from build123d import *

# Parameters (mm, degrees)
SKETCH1_R                = 7.5
BOSS_EXTRUDE1_DEPTH      = 8
M4_CLEARANCE_HOLE1_D     = 4.3
M4_CLEARANCE_HOLE1_DEPTH = 25
M4_CLEARANCE_HOLE1_TIP   = 1.291850331


with BuildPart() as part:
    # Sketch1 → Boss-Extrude1 (new body)
    with BuildSketch(Plane.XY):
        with BuildLine():
            Line((0.318181818, 17.497107199), (110.281818182, 15.497437805))
            ThreePointArc((110.281818182, 15.497437805), (125.5, 0), (110.281818182, -15.497437805))
            Line((110.281818182, -15.497437805), (0.318181818, -17.497107199))
            ThreePointArc((0.318181818, -17.497107199), (-17.5, 0), (0.318181818, 17.497107199))
        make_face()
        with Locations((110, 0)):
            Circle(SKETCH1_R, mode=Mode.SUBTRACT)
        with BuildLine():
            Line((35, 6.828401482), (35, -6.828401482))
            ThreePointArc((35, -6.828401482), (35.598701901, -8.255413618), (37.036363636, -8.828070876))
            Line((37.036363636, -8.828070876), (83.036363636, -7.991568964))
            ThreePointArc((83.036363636, -7.991568964), (84.427012136, -7.393197669), (85, -5.991899569))
            Line((85, -5.991899569), (85, 5.991899569))
            ThreePointArc((85, 5.991899569), (84.427012136, 7.393197669), (83.036363636, 7.991568964))
            Line((83.036363636, 7.991568964), (37.036363636, 8.828070876))
            ThreePointArc((37.036363636, 8.828070876), (35.598701901, 8.255413618), (35, 6.828401482))
        make_face(mode=Mode.SUBTRACT)
    extrude(amount=BOSS_EXTRUDE1_DEPTH)

    # M4 Clearance Hole1
    with Locations(Plane.XY.offset(8)):
        with Locations((12.124355653, 7), (0, 14), (-12.124355653, 7), (-12.124355653, -7), (0, -14), (12.124355653, -7)):
            Hole(M4_CLEARANCE_HOLE1_D / 2, depth=M4_CLEARANCE_HOLE1_DEPTH)
            with Locations((0, 0, -(M4_CLEARANCE_HOLE1_DEPTH + M4_CLEARANCE_HOLE1_TIP / 2))):  # 118° drill point
                Cone(0, M4_CLEARANCE_HOLE1_D / 2, M4_CLEARANCE_HOLE1_TIP, mode=Mode.SUBTRACT)


solid = part.part
Could you check a few things on this model? Use its own coordinates, in mm. A direction names the side the tool comes from. Give positions to 0.01 mm unless a question says otherwise; leave off trailing zeros. Order: outer loops, then holes, each group sorted by start corner. A loop starts at its lowest first (then second) coordinate and runs counter-clockwise, first axis right, second up.
1. For faces 5 (the flat face through (55, -11, 0)), 6 (the flat face through (35, 0, 4)), which set-ups out of +Z, -Z, +X, -X, +Y, -Y let a thin tool reach every point of the face, with its end or its side?
2. I need wall thicknesses on L1, parallel to Y at x = 14, z = 5; L2, parallel to Y at x = 13, z = 6; L3, parallel to X at y = -1, z = 2. Which ranges of each line are inside material? Lowest first, please.
3. We'd pull the mould along Y, two halves only. Please class faces 1 (the flat face through (55, -11, 8)), 2 (the cylindrical face through (-11.84, -4.87, 3.94)), 3 (the cylindrical face through (-17.496, -0.389, 3.944)), 4 (the cylindrical face through (0.47, 11.9, 3.94)): pulls with the +Y half, pulls with the -Y half, needs draft (parallel to the pull), parting line crosses it, or undercut.
4. Suppose I cut it at D-D (y = -14). List the corners of the cut face in (x, z) for me.
5. Will these pins go through, and if not, where does the flat tip stop? P1, Ø1, axis at x = 16, z = 6, coming from the +Y side; P2, Ø4, axis at y = 10.5, z = 1.5, coming from the +X side.
6. Suppose I cut it at B-B (z = 5.25). Give the number of separate pieces and of enclosed holes in the cut face, plus the area to 3 significant figures.
7. Suppose I cut it at C-C (x = 76). List the corners of the cut face in (y, z) for me, plus the area to 3 significant figures.
8. Suppose I cut it at A-A (y = 0). List the corners of the cut face in (x, z) for me.
Solved:
1. face 5: -Z, +X, -X, +Y, -Y
1. face 6: +Z, -Z
2. L1: y = -17.25 to -8.05, -5.95 to 5.95, 8.05 to 17.25
2. L2: y = -17.27 to -8.96, -5.04 to 5.04, 8.96 to 17.27
2. L3: x = -17.47 to 35, 85 to 102.57, 117.43 to 125.47
3. face 1: needs draft
3. face 2: undercut
3. face 3: parting line crosses it
3. face 4: undercut
4. outline: (-10.5, 0) - (-2.15, 0) - (-2.15, 8) - (-10.5, 8) - close; (2.15, 0) - (116.65, 0) - (116.65, 8) - (2.15, 8) - close
5. P1: stops at y = 17.22
5. P2: stops at x = 122.96
6. separate pieces: 1
6. enclosed holes: 8
6. area: 3,390 mm2
7. outline: (-16.12, 0) - (-8.12, 0) - (-8.12, 8) - (-16.12, 8) - close; (8.12, 0) - (16.12, 0) - (16.12, 8) - (8.12, 8) - close
7. area: 128 mm2
8. outline: (-17.5, 0) - (35, 0) - (35, 8) - (-17.5, 8) - close; (85, 0) - (102.5, 0) - (102.5, 8) - (85, 8) - close; (117.5, 0) - (125.5, 0) - (125.5, 8) - (117.5, 8) - close
